The model under review builds one solid part; all positions refer to its coordinate system, in mm. Face numbers are marked on the shaded views. Round coordinates to 2 decimals unless told otherwise and drop trailing zeros. Write each loop counter-clockwise with the first axis right and the second up, starting at its lowest first coordinate (ties: lowest second). Pieces come first, ordered by that corner, then holes. Notation, with made-up numbers: (56.25, 26.5) - (69.25, 26.5) arc R15 cw to (69.25, 51.5) - close; hole circle Ø4 at (49.5, 58.5). An arc over 180 degrees is marked (long way). Use one line per item in the form item = value.
from build123d import *

# Parameters (mm, degrees)
SKETCH1_W           = 40
SKETCH1_H           = 20
BOSS_EXTRUDE1_DEPTH = 10
SKETCH2_R           = 4
CUT_EXTRUDE1_DEPTH  = 5


with BuildPart() as part:
    # Sketch1 → Boss-Extrude1 (new, symmetric)
    with BuildSketch(Plane.XY):
        with Locations((20, 10)):
            Rectangle(SKETCH1_W, SKETCH1_H)
    extrude(amount=BOSS_EXTRUDE1_DEPTH, both=True)

    # Sketch2 → Cut-Extrude1 (cut)
    with BuildSketch(Plane.XY):
        with Locations((20, 10)):
            Circle(SKETCH2_R)
    extrude(amount=CUT_EXTRUDE1_DEPTH, mode=Mode.SUBTRACT)


solid = part.part
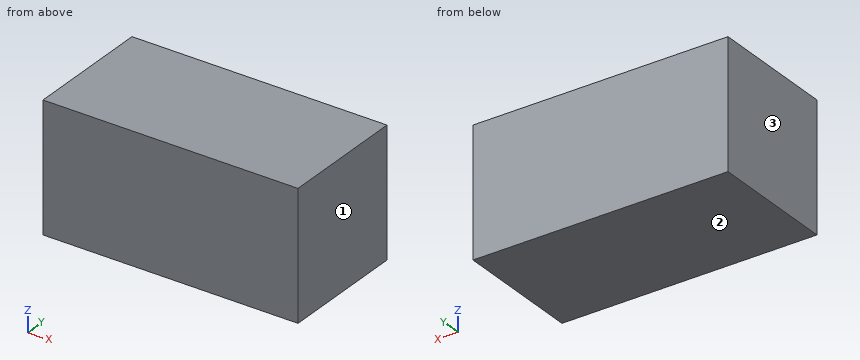
(1) Add section A-A on y = 10. Write out the cut boundary in (x, z).
Geometry results:
outline = (0, -10) - (40, -10) - (40, 10) - (0, 10) - close; hole (16, 0) - (24, 0) - (24, 5) - (16, 5) - close
(2) To check wall thickness, follow L1, parallel to Y at x = 20, z = 3.65; L2, parallel to Z at x = 18, y = 10.25. State the ranges of each line that lie inside material, in increasing order.
Geometry results:
L1 = 0 to 6, 14 to 20
L2 = -10 to 0, 5 to 10
(3) Insertion check: P1, Ø6, axis at x = 13, z = -1.5, coming from the -Y side. The pin has a flat end and moves straight along its axis. Give the tip position at first contact, or say it passes through.
Geometry results:
P1 = 0
(4) Add section B-B on x = 20. Write out the cut boundary in (y, z), then the cut area to 3 significant figures.
Geometry results:
outline = (0, -10) - (20, -10) - (20, 10) - (0, 10) - close; hole (6, 0) - (14, 0) - (14, 5) - (6, 5) - close
area = 360 mm2
(5) The part is to be moulded in two halves that separate along X. For the marked faces 1, 2 and 3, say which applies: +X half, -X half, draft (parallel to the pull), parting line (faces both ways), or undercut.
Geometry results:
face_1 = +X half
face_2 = draft
face_3 = -X half
